Here's how the part is built. I have some questions about the finished solid (model axes, mm). Face numbers are marked on the shaded views. A direction names the side the tool comes from. Coordinates: 2 decimals unless noted, no trailing zeros. Write each loop counter-clockwise with the first axis right and the second up, starting at its lowest first coordinate (ties: lowest second). Pieces come first, ordered by that corner, then holes.
Item 1: If we section it at A-A (z = -5): Please give me the cut outline in (x, y), then the cut area to 3 significant figures.
Item 2: I'm going to push flat-ended pins straight in: pin 1 Ø5 at (y, z) = (-8, 4.5) entering from +X; pin 2 Ø6 at (y, z) = (-11.5, -3.5) entering from -X; pin 3 Ø2 at (y, z) = (-1.5, 13.5) entering from -X; pin 4 Ø14.5 at (x, z) = (0, 0) entering from +Y. Where does each tip first touch, or does it pass through?
Item 3: We'd pull the mould along Z, two halves only. Please class the marked faces 3, 4 and 5: +Z half, -Z half, draft (parallel to the pull), parting line (faces both ways), or undercut.
Item 4: If we section it at B-B (x = -3): Please give me the cut outline in (y, z), then the cut area to 3 significant figures.
Item 5: If we section it at C-C (y = -11): Count the separate pieces of the cut face and the enclosed holes in it, then the cut area to 3 significant figures.
Item 6: If I drill on line 1 (Z direction, x = 2, y = -9); line 2 (X direction, y = -3.5, z = -2.5); line 3 (X direction, y = -8.5, z = 7), over which ranges is the centre line in solid material (lowest first)?
Item 7: For the marked faces 1 and 2, which set-ups out of +Z, -Z, +X, -X, +Y, -Y let a thin tool reach every point of the face, with its end or its side?
Item 8: If we section it at D-D (x = -18): Please give me the cut outline in (y, z).
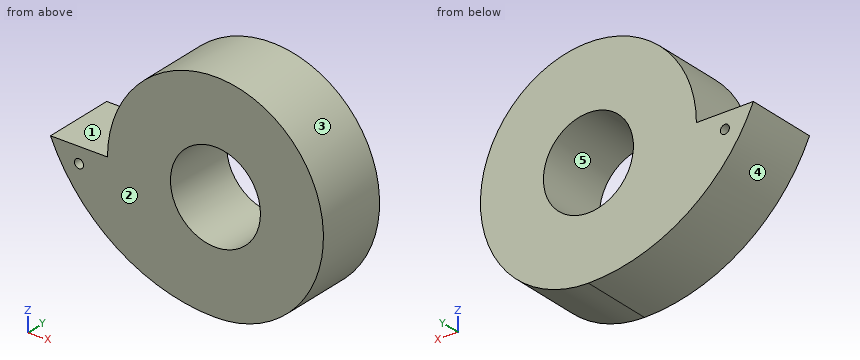
from build123d import *

# Parameters (mm, degrees)
F0_R           = 12.7
F0_R_2         = 7.9375
F1_DEPTH       = 12.7
F3_D           = 1.5875
F3_DEPTH       = 25.4
F3_CBORE_D     = 1.5875
F3_CBORE_DEPTH = 6.35
F3_TIP         = 0.4769331164


with BuildPart() as f1:
    # F0 (on Front) → F1 (new body)
    with BuildSketch(Plane.XZ):
        with BuildLine():
            ThreePointArc((0, -19.05), (13.4703841816, -13.4703841816), (19.05, 0))
            ThreePointArc((19.05, 0), (0, 19.05), (-19.05, 0))
            ThreePointArc((-19.05, 0), (-13.4703841816, -13.4703841816), (0, -19.05))
        make_face()
        Circle(F0_R, mode=Mode.SUBTRACT)
        Circle(F0_R)
        Circle(F0_R_2, mode=Mode.SUBTRACT)
        with BuildLine():
            ThreePointArc((0, -19.05), (-13.4703841816, -13.4703841816), (-19.05, 0))
            Line((-19.05, 0), (-29.099355663, 0))
            ThreePointArc((-29.099355663, 0), (-17.3901912008, -13.8639558425), (0, -19.05))
        make_face()
    extrude(amount=F1_DEPTH)

    # F3
    with Locations(Plane.XZ.offset(12.7)):
        with Locations((-24.0746778315, -2.738931682)):
            CounterBoreHole(F3_D / 2, F3_CBORE_D / 2, F3_CBORE_DEPTH, depth=F3_DEPTH)
            with Locations((0, 0, -(F3_DEPTH + F3_TIP / 2))):  # 118° drill point
                Cone(0, F3_D / 2, F3_TIP, mode=Mode.SUBTRACT)


solid = f1.part
Answer list:
1. outline: (-26.36, -12.7) - (-6.16, -12.7) - (-6.16, 0) - (-26.36, 0) - close; (6.16, -12.7) - (18.38, -12.7) - (18.38, 0) - (6.16, 0) - close
1. area: 412 mm2
2. pin 1: stops at x = 18.94
2. pin 2: stops at x = -28.88
2. pin 3: stops at x = -14.38
2. pin 4: passes through
3. face 3: parting line
3. face 4: -Z half
3. face 5: undercut
4. outline: (-12.7, -18.91) - (0, -18.91) - (0, -7.35) - (-12.7, -7.35) - close; (-12.7, 7.35) - (0, 7.35) - (0, 18.81) - (-12.7, 18.81) - close
4. area: 292 mm2
5. separate pieces: 1
5. enclosed holes: 2
5. area: 1,050 mm2
6. line 1: z = -18.94 to -7.68, 7.68 to 18.94
6. line 2: x = -27.88 to -24.83, -23.32 to -7.53, 7.53 to 18.89
6. line 3: x = -17.72 to -3.74, 3.74 to 17.72
7. face 1: +Z, -X, +Y, -Y
7. face 2: +Z, -Z, +X, -X, -Y
8. outline: (-12.7, -13.45) - (0, -13.45) - (0, 6.24) - (-12.7, 6.24) - close
